Design review of the part built by this model. Coordinates are the model's own, in mm. Face numbers are marked on the shaded views. A direction names the side the tool comes from. Give positions to 0.01 mm unless a question says otherwise; leave off trailing zeros. Write each loop counter-clockwise with the first axis right and the second up, starting at its lowest first coordinate (ties: lowest second). Pieces come first, ordered by that corner, then holes. Notation, with made-up numbers: (-33, -39) -> (-11, -39) arc R12 cw to (-11, -17) -> close; hole circle Ø3 at (28, -28.75). An arc over 180 degrees is marked (long way). Answer as a JSON object with one key per item and string values.
```python
from build123d import *

# Parameters (mm, degrees)
EXTRUDE1_DEPTH = 40
SKETCH2_W      = 20
SKETCH2_H      = 20
EXTRUDE2_DEPTH = 52.923019943
SKETCH3_R      = 1.5
EXTRUDE3_DEPTH = 52.923019943
SKETCH4_R      = 1.5
EXTRUDE4_DEPTH = 47.861498055
EXTRUDE5_DEPTH = 9.5


with BuildPart() as part:
    # Sketch1 → Extrude1 (new body)
    with BuildSketch(Plane(origin=(0, 0, 0), x_dir=(0, 0, -1), z_dir=(1, 0, 0))):
        Polygon((0, 0), (-14, 0), (-4, 30), (0, 30), align=None)
    extrude(amount=-EXTRUDE1_DEPTH)

    # Sketch2 → Extrude2 (cut, through all)
    with BuildSketch(Plane(origin=(0, 0, 0), x_dir=(-1, 0, 0), z_dir=(0, 0, -1))):
        with Locations((20, 20)):
            Rectangle(SKETCH2_W, SKETCH2_H)
    extrude(amount=-EXTRUDE2_DEPTH, mode=Mode.SUBTRACT)

    # Sketch3 → Extrude3 (cut, through all)
    with BuildSketch(Plane(origin=(0, 0, 0), x_dir=(-1, 0, 0), z_dir=(0, 0, -1))):
        with Locations(Location((5, 20, 0), (0, 0, 90))):
            Circle(SKETCH3_R)
        with Locations(Location((35, 20, 0), (0, 0, 90))):
            Circle(SKETCH3_R)
    extrude(amount=-EXTRUDE3_DEPTH, mode=Mode.SUBTRACT)

    # Sketch4 → Extrude4 (cut, through all)
    with BuildSketch(Plane(origin=(0, 10, 0), x_dir=(1, 0, 0), z_dir=(0, 1, 0))):
        with Locations(Location((-24.95, -3.95, 0), (0, 0, 270))):
            Circle(SKETCH4_R)
        with Locations(Location((-15.05, -3.95, 0), (0, 0, 90))):
            Circle(SKETCH4_R)
    extrude(amount=-EXTRUDE4_DEPTH, mode=Mode.SUBTRACT)

    # Sketch8 → Extrude5 (cut)
    with BuildSketch(Plane(origin=(0, 0, 14), x_dir=(-1, 0, 0), z_dir=(0, 0, -1))):
        Polygon((6.58771324, 17.25), (8.175426481, 20), (6.58771324, 22.75), (3.41228676, 22.75), (1.824573519, 20), (3.41228676, 17.25), align=None)
        Polygon((36.58771324, 17.25), (33.41228676, 17.25), (31.824573519, 20), (33.41228676, 22.75), (36.58771324, 22.75), (38.175426481, 20), align=None)
    extrude(amount=EXTRUDE5_DEPTH, mode=Mode.SUBTRACT)


solid = part.part
```
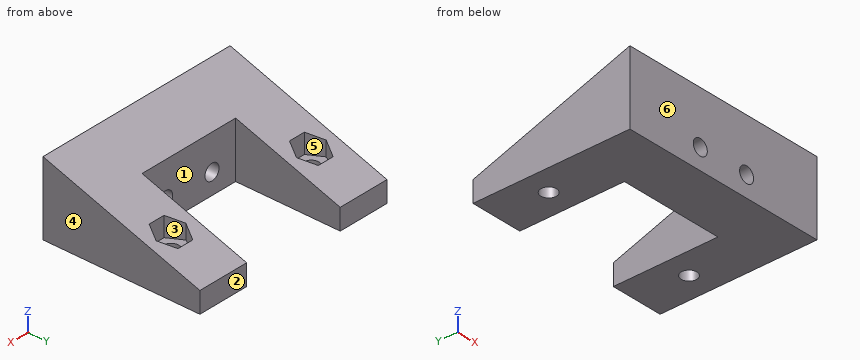
(1) The part is to be moulded in two halves that separate along Y. For the marked faces 3, 4, 5 and 6, say which applies: +Y half, -Y half, draft (parallel to the pull), parting line (faces both ways), or undercut.
Here are the results:
{"face 3": "undercut", "face 4": "draft", "face 5": "undercut", "face 6": "-Y half"}
(2) For line 1 along X through (y, z) = (20, 1.2); line 2 along X through (y, z) = (6.25, 3.95); line 3 along X through (y, z) = (12, 2.5), list the stretches that pass through material, from the lowest coordinate up.
Here are the results:
{"line 1": "x = -40 to -36.5, -33.5 to -30, -10 to -6.5, -3.5 to 0", "line 2": "x = -40 to -26.45, -23.45 to -16.55, -13.55 to 0", "line 3": "x = -40 to -30, -10 to 0"}
(3) We need section D-D, the plane x = -24.95. State the section outline as (y, z) points.
Here are the results:
{"outline": "(0, 0) -> (10, 0) -> (10, 2.45) -> (0, 2.45) -> close; (0, 5.45) -> (10, 5.45) -> (10, 10.67) -> (0, 14) -> close"}
(4) We need section B-B, the plane y = 14. State the section outline as (x, z) points.
Here are the results:
{"outline": "(-40, 0) -> (-30, 0) -> (-30, 9.33) -> (-40, 9.33) -> close; (-10, 0) -> (0, 0) -> (0, 9.33) -> (-10, 9.33) -> close"}
(5) We need section C-C, the plane z = 8.75. State the section outline as (x, y) points, then the cut area to 3 significant figures.
Here are the results:
{"outline": "(-40, 0) -> (0, 0) -> (0, 15.75) -> (-10, 15.75) -> (-10, 10) -> (-30, 10) -> (-30, 15.75) -> (-40, 15.75) -> close", "area": "515 mm²"}
(6) We need section A-A, the plane x = -35. State the section outline as (y, z) points, then the cut area to 3 significant figures.
Here are the results:
{"outline": "(0, 0) -> (18.5, 0) -> (18.5, 4.5) -> (17.25, 4.5) -> (17.25, 8.25) -> (0, 14) -> close; (21.5, 0) -> (30, 0) -> (30, 4) -> (22.75, 6.42) -> (22.75, 4.5) -> (21.5, 4.5) -> close", "area": "241 mm²"}
(7) For the marked faces 1 and 2, list the 3-axis set-ups (+Z, -Z, +X, -X, +Y, -Y) from which the entire face can be reached by the end or side of a thin tool; tool diameter is ignored.
Here are the results:
{"face 1": "+Z, -Z, +Y", "face 2": "+Z, -Z, +X, -X, +Y"}
(8) Clearance check with flat-ended pins moving along their axes: pin 1 (5.5 mm diameter, centred on x = -19.5, z = 3.5, fed in from +Y); pin 2 (3 mm diameter, centred on x = -4, y = 19, fed in from +Z); pin 3 (6 mm diameter, centred on x = -34, y = 21, fed in from +Z); pin 4 (2.5 mm diameter, centred on x = -5, y = 20, fed in from +Z). State where each tip first meets the part, or that it passes through.
Here are the results:
{"pin 1": "stops at y = 10", "pin 2": "stops at z = 8.06", "pin 3": "stops at z = 7.92", "pin 4": "passes through"}
